Can you work these out from the model? Positions are in its coordinate system, mm. Coordinates: 2 decimals unless noted, no trailing zeros. Order: outer loops, then holes, each group sorted by start corner. A loop starts at its lowest first (then second) coordinate and runs counter-clockwise, first axis right, second up. Notation, with made-up numbers: (47.5, 42) - (57.5, 42) arc R20 ccw to (57.5, 47) - close; hole circle Ø11 at (88.5, 62). An arc over 180 degrees is marked (long way). Use a Markdown table: item, result. Add a question column.
(1) If I drill on L1, parallel to Y at x = 0, z = 1; L2, parallel to Y at x = -5, z = 2.3; L3, parallel to X at y = -8.5, z = 0.9, over which ranges is the centre line in solid material (lowest first)? Write a range as [from, to].
(2) We'd pull the mould along X, two halves only. Please class faces 1 (the flat face through (16, 2, 0)), 2 (the flat face through (15.073, -14.415, 1.479)), 3 (the cylindrical face through (0.69, -1.33, 1.48)): pulls with the +X half, pulls with the -X half, needs draft (parallel to the pull), parting line crosses it, or undercut.
(3) I want a section at A-A (y = 0). List the corners of the cut face in (x, z) for me.
(4) For pin 1 Ø1.5 at (x, z) = (20.5, 2.5) entering from -Y; pin 2 Ø1.5 at (x, z) = (3.5, 1.5) entering from +Y; pin 3 Ø1.5 at (x, z) = (10.5, 0.5) entering from +Y, each with a flat end and sliding along its axis, tell me the tip position at first contact or that it passes through.
(5) I want a section at D-D (x = 13). List the corners of the cut face in (y, z) for me.
(6) I want a section at C-C (x = 0). List the corners of the cut face in (y, z) for me, and give its area (3 significant figures).
(7) I want a section at B-B (z = 1.15). List the corners of the cut face in (x, y) for me.
```python
from build123d import *

# Parameters (mm, degrees)
MODEL_R                 = 1.500000302
SALIENTE_EXTRUIR1_DEPTH = 3


with BuildPart() as part:
    # Model → Saliente-Extruir1 (new body)
    with BuildSketch(Plane.XY):
        with BuildLine():
            Line((33.092598302, 20.364675113), (33.092598302, 33.261670113))
            Line((33.092598302, 33.261670113), (-5.597442698, 8.883616113))
            ThreePointArc((-5.597442698, 8.883616113), (-10.360174651, -1.707858659), (-2.449856698, -10.210200887))
            Line((-2.449856698, -10.210200887), (33.092598302, -18.738329887))
            Line((33.092598302, -18.738329887), (33.092598302, 20.364675113))
        make_face()
        Circle(MODEL_R, mode=Mode.SUBTRACT)
    extrude(amount=SALIENTE_EXTRUIR1_DEPTH)


solid = part.part
```
Answers follow:
| question | item | result |
|---|---|---|
| 1 | L1 | y = [-10.8, -1.5], [1.5, 12.41] |
| 1 | L2 | y = [-9.23, 9.26] |
| 1 | L3 | x = [-6.16, 33.09] |
| 2 | face 1 | needs draft |
| 2 | face 2 | pulls with the -X half |
| 2 | face 3 | undercut |
| 3 | outline | (-10.5, 0) - (-1.5, 0) - (-1.5, 3) - (-10.5, 3) - close; (1.5, 0) - (33.09, 0) - (33.09, 3) - (1.5, 3) - close |
| 4 | pin 1 | stops at y = -15.9 |
| 4 | pin 2 | stops at y = 15.09 |
| 4 | pin 3 | stops at y = 19.5 |
| 5 | outline | (-13.92, 0) - (20.6, 0) - (20.6, 3) - (-13.92, 3) - close |
| 6 | outline | (-10.8, 0) - (-1.5, 0) - (-1.5, 3) - (-10.8, 3) - close; (1.5, 0) - (12.41, 0) - (12.41, 3) - (1.5, 3) - close |
| 6 | area | 60.6 mm² |
| 7 | outline | (-5.6, 8.88) arc R10.5 ccw to (-2.45, -10.21) - (33.09, -18.74) - (33.09, 33.26) - close; hole circle Ø3 at (0, 0) |
